```python
from build123d import *

# Parameters (mm, degrees)
F1_DEPTH = 6.35
F4_DEPTH = 330.201
F6_DEPTH = 877.312735


with BuildPart() as f1:
    # F0 (on Front) → F1 (new body, symmetric)
    with BuildSketch(Plane.XZ):
        Polygon((206.782042, 184.344013), (-123.417958, 184.344013), (206.782042, -628.455987), align=None)
    extrude(amount=F1_DEPTH, both=True)

    # F3 (on face) → F4 (cut, through all)
    with BuildSketch(Plane.YZ.offset(206.782042)):
        Polygon((-6.35, 178.689609), (6.35, 184.344013), (-6.35, 184.344013), align=None)
    extrude(amount=-F4_DEPTH, mode=Mode.SUBTRACT)

    # F5 (on face) → F6 (cut, through all)
    with BuildSketch(Plane(origin=(-81.764245, 0, 201.265834), x_dir=(0.926467, 0, 0.376377), z_dir=(0.376377, 0, -0.926467))):
        Polygon((-44.959792, 6.350266), (-44.959792, -6.476734), (-42.813289, -6.476734), align=None)
    extrude(amount=F6_DEPTH, mode=Mode.SUBTRACT)


solid = f1.part
```
For this review, take the finished solid that the model builds, in its own axes (mm). Give positions to 0.01 mm unless a question says otherwise; leave off trailing zeros. Write each loop counter-clockwise with the first axis right and the second up, starting at its lowest first coordinate (ties: lowest second). Pieces come first, ordered by that corner, then holes.
Item 1: Take a section at C-C (y = 4). Give the boundary of the cut face in (x, z).
Item 2: Insertion check: P1, Ø6, axis at y = -2.5, z = 77.5, coming from the -X side; P2, Ø5, axis at x = 8.5, y = -1, coming from the +Z side. Each pin has a flat end and moves straight along its axis. Give the tip position at first contact, or say it passes through.
Item 3: Wall thickness on probe 1 along Z at (x, y) = (-3, 4.5); probe 2 along Z at (x, y) = (67, 2.25); probe 3 along X at (y, z) = (-3.25, -410): over which ranges is each line inside the solid? List them lowest first.
Established:
1. outline: (-121.12, 183.3) - (206.78, -623.85) - (206.78, 183.3) - close
2. P1: stops at x = -80.65
2. P2: stops at z = 182.18
3. probe 1: z = -107.25 to 183.52
3. probe 2: z = -280.55 to 182.52
3. probe 3: x = 118.59 to 206.78
